Autodesk Inventor part; units mm, degrees
ref_plane "YZ Plane" through (0, 0, 0) normal (1, 0, 0) x (0, 1, 0)
ref_plane "XZ Plane" through (0, 0, 0) normal (0, 1, 0) x (-1, 0, 0)
ref_plane "XY Plane" through (0, 0, 0) normal (0, 0, 1) x (1, 0, 0)
sketch "Sketch1" plane through (0, 0, 0) normal (0, 1, 0) x (-1, 0, 0)
  line L0 (0, 0) -> (53.34, 0)
  line L1 (53.34, 0) -> (53.34, -68.58)
  line L2 (53.34, -68.58) -> (0, -68.58)
  line L3 (0, -68.58) -> (0, 0)
  line L4 (53.34, -66) -> (0, -66) construction
  circle A0 centre (7.62, -66) radius 1.5
  circle A1 centre (35.56, -66) radius 1.5
  circle A2 centre (2.5, -14) radius 1.5
  line L5 (-5, -73.58) -> (58.34, -73.58)
  line L6 (58.34, -73.58) -> (58.34, 5)
  line L7 (58.34, 5) -> (-5, 5)
  line L8 (-5, 5) -> (-5, -73.58)
  dimension "d0" = 68.58
  dimension "d1" = 53.34
  dimension "d2" = 2.58
  dimension "d3" = 3
  dimension "d4" = 7.62
  dimension "d5" = 3
  dimension "d6" = 35.56
  dimension "d8" = 3
  dimension "d9" = 14
  dimension "d10" = 2.5
  dimension "d46" = 5
  dimension "d73" = 63.34
  dimension "d74" = 78.58
extrude "Extrusion4" add sketch "Sketch1" along normal blind 1 contours L0 L1 L2 L3 | L8 L7 L6 L5
sketch "Sketch5" plane through (0, 1, 0) normal (0, 1, 0) x (1, 0, 0)
  line L0 (5, -5) -> (0, -5)
  line L1 (0, -5) -> (0, 0)
  line L2 (0, 0) -> (5, 0)
  line L3 (5, 0) -> (5, -5)
  dimension "d49" = 5
  dimension "d50" = 5
extrude "Extrusion5" add sketch "Sketch5" along normal blind 7
ref_plane "Work Plane2" through (-26.67, 0, 5) normal (1, 0, 0) x (0, 0, -1)
mirror "Mirror2" about plane through (-26.67, 0, 5) normal (1, 0, 0) of "Extrusion5"
ref_plane "Work Plane3" through (-58.34, 0, -34.29) normal (0, 0, 1) x (1, 0, 0)
mirror "Mirror3" about plane through (-58.34, 0, -34.29) normal (0, 0, 1) of "Extrusion5", "Mirror2"
sketch "Sketch6" plane through (0, 1, 0) normal (0, 1, 0) x (1, 0, 0)
  line L0 (-51.17, 0.5) -> (-9.17, 0.5)
  line L1 (-9.17, 0.5) -> (-9.17, 62.5)
  line L2 (-9.17, 62.5) -> (-51.17, 62.5)
  line L3 (-51.17, 62.5) -> (-51.17, 0.5)
  line L4 (-52.17, 63.5) -> (-8.17, 63.5)
  line L5 (-8.17, 63.5) -> (-8.17, -0.5)
  line L6 (-8.17, -0.5) -> (-52.17, -0.5)
  line L7 (-52.17, -0.5) -> (-52.17, 63.5)
  line L8 (-52.17, 4.5) -> (-51.17, 4.5)
  line L9 (-47.17, 0.5) -> (-47.17, -0.5)
  line L10 (-47.17, 63.5) -> (-47.17, 62.5)
  line L11 (-51.17, 58.5) -> (-52.17, 58.5)
  line L12 (-13.17, 0.5) -> (-13.17, -0.5)
  line L13 (-9.17, 4.5) -> (-8.17, 4.5)
  line L14 (-9.17, 58.5) -> (-8.17, 58.5)
  line L15 (-13.17, 63.5) -> (-13.17, 62.5)
  point P0 (0, 0)
  point P1 (-30.17, 0.5)
  dimension "d34" = 42
  dimension "d35" = 62
  dimension "d39" = 1
  dimension "d40" = 5
  dimension "d41" = 5
  dimension "d44" = 5
  dimension "d45" = 5
  dimension "d62" = 5
  dimension "d63" = 5
  dimension "d64" = 5
  dimension "d65" = 5
sketch "Sketch7" plane through (0, 8, 0) normal (0, 1, 0) x (1, 0, 0)
  line L0 (0, 0) -> (0, -5)
  line L1 (0, -5) -> (5, -5)
  line L2 (5, -5) -> (5, 0)
  line L3 (5, 0) -> (0, 0)
  circle A0 centre (2.5, -2.5) radius 1
  dimension "d53" = 5
  dimension "d54" = 2
hole "Hole1" [suppressed]
mirror "Mirror8" [suppressed]
mirror "Mirror9" [suppressed]
extrude "Extrusion8" add sketch "Sketch6" along normal blind 7 contours L0 L1 L13 L5 L6 L12 | L11 L7 L4 L10 L2 L3 | L1 L2 L15 L4 L5 L14
sketch "Sketch8" plane through (0, 1, 0) normal (0, 1, 0) x (1, 0, 0)
  line L0 (-58.34, 73.58) -> (-58.34, -5)
  line L1 (-58.34, 2) -> (-53.34, 2)
  line L2 (-53.34, 2) -> (-53.34, 12)
  line L3 (-53.34, 12) -> (-58.34, 12)
  line L4 (-58.34, 12) -> (-58.34, 2)
  line L5 (-58.34, 0) -> (-53.34, 0)
  point P0 (0, 0)
  dimension "d68" = 5
  dimension "d69" = 10
  dimension "d70" = 2
extrude "Extrusion9" cut sketch "Sketch8" against normal blind 1
properties part number "sensor3"
CAD build for the part. Positions are in the model's coordinates, mm. A direction names the side the tool comes from. Coordinates: 2 decimals unless noted, no trailing zeros. Write each loop counter-clockwise with the first axis right and the second up, starting at its lowest first coordinate (ties: lowest second). Pieces come first, ordered by that corner, then holes. Notation, with made-up numbers: (-35.75, 40) -> (13.25, 40) arc R19 ccw to (13.25, 57) -> close; hole circle Ø1 at (-38, -10.5). An arc over 180 degrees is marked (long way). Use CSV: the item, a comma, the result in double quotes. Start each with the question number.
Item 1: Two-plate mould, pull along Z, no slides. Class faces 1 (the flat face through (-50, 4, -63.5)), 2 (the flat face through (2, 4, 0)), 3 (the flat face through (2, 8, 2)): +Z half, -Z half, draft (parallel to the pull), parting line (faces both ways), or undercut.
Item 2: Band-saw the part on B-B, the plane y = 4. Give the number of separate pieces and of enclosed holes in the cut face, plus the area to 3 significant figures.
Item 3: Band-saw the part on A-A, the plane z = -66. Write the cut outline in (x, y).
Item 4: Band-saw the part on C-C, the plane z = -14. Write the cut outline in (x, y).
Item 5: Drop flat-ended pins along their axis: P1, Ø2, axis at x = -50, z = -39.5, coming from the -Y side; P2, Ø4, axis at y = 6, z = -61.5, coming from the +X side; P3, Ø1, axis at x = -41, z = -10.5, coming from the +Y side; P4, Ø4.5, axis at x = -10.5, y = 4.5, coming from the -Z side. Give the stop position or say it passes through.
Item 6: Tool access for faces 4 (the flat face through (-11, 4, -63.5)), 5 (the flat face through (-9.17, 4, -2)), 6 (the flat face through (-53.34, 4, 2)), 7 (the flat face through (-9.17, 4, -60)), 8 (the flat face through (-49, 4, -62.5)): list every direction of +Z, -Z, +X, -X, +Y, -Y with a clear straight run to the whole face (end or side of a thin tool).
Item 7: Wall check: probe 1 along X at (y, z) = (0.4, -66); probe 2 along Z at (x, y) = (1, 7.25); probe 3 along Z at (x, y) = (-7.62, 0.3). Give the ranges that are in metal, low to high.
Item 8: Band-saw the part on D-D, the plane x = -35.56. Write the cut outline in (y, z), plus the area to 3 significant figures.
Response values:
1,face 1,"-Z half"
1,face 2,"undercut"
1,face 3,"draft"
2,separate pieces,"7"
2,enclosed holes,"0"
2,area,"127 mm2"
3,outline,"(-58.34, 0) -> (-37.06, 0) -> (-37.06, 1) -> (-58.34, 1) -> close; (-34.06, 0) -> (-9.12, 0) -> (-9.12, 1) -> (-34.06, 1) -> close; (-6.12, 0) -> (5, 0) -> (5, 1) -> (-6.12, 1) -> close"
4,outline,"(-58.34, 0) -> (-4, 0) -> (-4, 1) -> (-58.34, 1) -> close; (-1, 0) -> (5, 0) -> (5, 1) -> (-1, 1) -> close"
5,P1,"stops at y = 0"
5,P2,"stops at x = -8.17"
5,P3,"stops at y = 1"
5,P4,"stops at z = -63.5"
6,face 4,"-Z, +X, -X, +Y"
6,face 5,"-X, +Y"
6,face 6,"+Z, -Z, +Y"
6,face 7,"+Y"
6,face 8,"+Z, +Y"
7,probe 1,"x = -58.34 to -37.06, -34.06 to -9.12, -6.12 to 5"
7,probe 2,"z = -73.58 to -68.58, 0 to 5"
7,probe 3,"z = -73.58 to -67.5, -64.5 to 5"
8,outline,"(0, -73.58) -> (1, -73.58) -> (1, -67.5) -> (0, -67.5) -> close; (0, -64.5) -> (1, -64.5) -> (1, 5) -> (0, 5) -> close"
8,area,"75.6 mm2"
